from build123d import *

# Parameters (mm, degrees)
BOSS_EXTRUDE1_DEPTH = 1.9
SKETCH5_W           = 2.15
SKETCH5_H           = 30
SKETCH4_W           = 2.15
SKETCH4_H           = 30
SKETCH6_R           = 1.5
CUT_EXTRUDE1_DEPTH  = 29


with BuildPart() as part:
    # Sketch2 → Boss-Extrude1 (new body)
    with BuildSketch(Plane.XY):
        with BuildLine():
            Line((-20.5, -0.95), (-13.5, -0.95))
            ThreePointArc((-13.5, -0.95), (-12.121141777, -0.378858223), (-11.55, 1))
            Line((-11.55, 1), (-11.55, 7))
            ThreePointArc((-11.55, 7), (-11, 7.55), (-10.45, 7))
            Line((-10.45, 7), (-10.45, 0))
            Line((-10.45, 0), (-10.45, -7))
            ThreePointArc((-10.45, -7), (-8, -9.45), (-5.55, -7))
            Line((-5.55, -7), (-5.55, 0))
            Line((-5.55, 0), (-5.55, 7))
            ThreePointArc((-5.55, 7), (-5, 7.55), (-4.45, 7))
            Line((-4.45, 7), (-4.45, 0))
            Line((-4.45, 0), (-4.45, -7))
            ThreePointArc((-4.45, -7), (-2, -9.45), (0.45, -7))
            Line((0.45, -7), (0.45, 0))
            Line((0.45, 0), (0.45, 7))
            ThreePointArc((0.45, 7), (1, 7.55), (1.55, 7))
            Line((1.55, 7), (1.55, 0))
            Line((1.55, 0), (1.55, -7))
            ThreePointArc((1.55, -7), (4, -9.45), (6.45, -7))
            Line((6.45, -7), (6.45, -1))
            ThreePointArc((6.45, -1), (6.464644661, -0.964644661), (6.5, -0.95))
            Line((6.5, -0.95), (13.5, -0.95))
            ThreePointArc((13.5, -0.95), (14.45, 0), (13.5, 0.95))
            Line((13.5, 0.95), (6.5, 0.95))
            ThreePointArc((6.5, 0.95), (5.121141777, 0.378858223), (4.55, -1))
            Line((4.55, -1), (4.55, -7))
            ThreePointArc((4.55, -7), (4, -7.55), (3.45, -7))
            Line((3.45, -7), (3.45, 0))
            Line((3.45, 0), (3.45, 7))
            ThreePointArc((3.45, 7), (1, 9.45), (-1.45, 7))
            Line((-1.45, 7), (-1.45, 0))
            Line((-1.45, 0), (-1.45, -7))
            ThreePointArc((-1.45, -7), (-2, -7.55), (-2.55, -7))
            Line((-2.55, -7), (-2.55, 0))
            Line((-2.55, 0), (-2.55, 7))
            ThreePointArc((-2.55, 7), (-5, 9.45), (-7.45, 7))
            Line((-7.45, 7), (-7.45, 0))
            Line((-7.45, 0), (-7.45, -7))
            ThreePointArc((-7.45, -7), (-8, -7.55), (-8.55, -7))
            Line((-8.55, -7), (-8.55, 0))
            Line((-8.55, 0), (-8.55, 7))
            ThreePointArc((-8.55, 7), (-11, 9.45), (-13.45, 7))
            Line((-13.45, 7), (-13.45, 1))
            ThreePointArc((-13.45, 1), (-13.464644661, 0.964644661), (-13.5, 0.95))
            Line((-13.5, 0.95), (-20.5, 0.95))
            ThreePointArc((-20.5, 0.95), (-21.45, 0), (-20.5, -0.95))
        make_face()
    extrude(amount=BOSS_EXTRUDE1_DEPTH)

    # Sketch5 → Revolve1 (revolve)
    with BuildSketch(Plane(origin=(0, 0, 0), x_dir=(1, 0, 0), z_dir=(0, 1, 0))):
        with Locations((-21.575, 13.1)):
            Rectangle(SKETCH5_W, SKETCH5_H)
    revolve(axis=Axis((-20.5, 0, -28.1), (0, 0, 1)))

    # Sketch4 → Revolve2 (revolve)
    with BuildSketch(Plane(origin=(0, 0, 0), x_dir=(1, 0, 0), z_dir=(0, 1, 0))):
        with Locations((14.575, 13.1)):
            Rectangle(SKETCH4_W, SKETCH4_H)
    revolve(axis=Axis((13.5, 0, 1.9), (0, 0, -1)))

    # Sketch6 → Cut-Extrude1 (cut)
    with BuildSketch(Plane(origin=(0, 0, -28.1), x_dir=(-1, 0, 0), z_dir=(0, 0, -1))):
        with Locations((-13.5, 0)):
            Circle(SKETCH6_R)
        with Locations((20.5, 0)):
            Circle(SKETCH6_R)
    extrude(amount=-CUT_EXTRUDE1_DEPTH, mode=Mode.SUBTRACT)


solid = part.part
For this review, take the finished solid that the model builds, in its own axes (mm). A direction names the side the tool comes from. Round coordinates to 2 decimals unless told otherwise and drop trailing zeros. Loops run counter-clockwise (first coordinate to the right, second up) from the corner with the lowest first, then second, coordinate; pieces in that order, holes last. Notation, with made-up numbers: (-22.5, -37.75) - (-3.5, -37.75) arc R13 ccw to (-3.5, -31.75) - close; hole circle Ø4 at (47, 20.25). An arc over 180 degrees is marked (long way). One line per question, with ' | ' between items.
Q1. Take a section at C-C (x = -20.5). Give the boundary of the cut face in (y, z).
Taken from the geometry:
outline: (-2.15, -28.1) - (-1.5, -28.1) - (-1.5, 0.9) - (1.5, 0.9) - (1.5, -28.1) - (2.15, -28.1) - (2.15, 1.9) - (-2.15, 1.9) - close
Q2. For pin 1 (0.6 mm diameter, centred on y = -1, z = 1, fed in from +X); pin 2 (1.5 mm diameter, centred on x = -16, z = 1, fed in from -Y); pin 3 (0.6 mm diameter, centred on y = -4.5, z = 0.5, fed in from +X), all flat-tipped, find the tip position at first contact; note any pin that passes through.
Taken from the geometry:
pin 1: stops at x = 15.53 | pin 2: stops at y = -0.95 | pin 3: stops at x = 6.45
Q3. Take a section at B-B (z = -12.25). Give the boundary of the cut face in (x, y).
Taken from the geometry:
outline: circle Ø4.3 at (-20.5, 0); circle Ø4.3 at (13.5, 0); hole circle Ø3 at (-20.5, 0); hole circle Ø3 at (13.5, 0)
Q4. For line 1 along Y through (x, z) = (13.5, -22); line 2 along Z through (x, y) = (-9.5, -6.5); line 3 along Y through (x, z) = (-14.5, 0.75), list the stretches that pass through material, from the lowest coordinate up. Write a range as [from, to].
Taken from the geometry:
line 1: y = [-2.15, -1.5], [1.5, 2.15] | line 2: z = [0, 1.9] | line 3: y = [-0.95, 0.95]
Q5. Take a section at A-A (y = -6.5). Give the boundary of the cut face in (x, z).
Taken from the geometry:
outline: (-10.45, 0) - (-8.55, 0) - (-8.55, 1.9) - (-10.45, 1.9) - close; (-7.45, 0) - (-5.55, 0) - (-5.55, 1.9) - (-7.45, 1.9) - close; (-4.45, 0) - (-2.55, 0) - (-2.55, 1.9) - (-4.45, 1.9) - close; (-1.45, 0) - (0.45, 0) - (0.45, 1.9) - (-1.45, 1.9) - close; (1.55, 0) - (3.45, 0) - (3.45, 1.9) - (1.55, 1.9) - close; (4.55, 0) - (6.45, 0) - (6.45, 1.9) - (4.55, 1.9) - close
Q6. Take a section at D-D (y = 8). Give the boundary of the cut face in (x, z).
Taken from the geometry:
outline: (-13.24, 0) - (-8.76, 0) - (-8.76, 1.9) - (-13.24, 1.9) - close; (-7.24, 0) - (-2.76, 0) - (-2.76, 1.9) - (-7.24, 1.9) - close; (-1.24, 0) - (3.24, 0) - (3.24, 1.9) - (-1.24, 1.9) - close
Q7. Tool access review of faces 1 (the flat face through (-20, 0, 0.9)), 2 (the cylindrical face through (5.136, 0.394, 0.937)), 3 (the cylindrical face through (-12.136, -0.394, 0.937)): name each direction out of +Z, -Z, +X, -X, +Y, -Y from which nothing blocks a thin tool from reaching the whole face with its end or side.
Taken from the geometry:
face 1: -Z | face 2: +Z, -Z, +Y | face 3: +Z, -Z, -Y
